Could you check a few things on this model? Use its own coordinates, in mm. A direction names the side the tool comes from. Coordinates: 2 decimals unless noted, no trailing zeros. Loops run counter-clockwise (first coordinate to the right, second up) from the corner with the lowest first, then second, coordinate; pieces in that order, holes last. Notation, with made-up numbers: M 29.5,31 L 34.5,31 A20 cw 34.5,62 Z; hole C -17,0 d10. An arc over 180 degrees is marked long. Return JSON: item names as keys, results as strings. Group by question number.
from build123d import *
from build123d.topology import SkipClean

# Parameters (mm, degrees)
BOSS_EXTRU_1_DEPTH           = 18
ENL_V_MAT_EXTRU_1_DEPTH      = 34.301651611
ENL_V_MAT_EXTRU_1_DEPTH_BACK = 34.301651611
ESQUISSE2_R                  = 2.85
ENL_V_MAT_EXTRU_2_DEPTH      = 34.301651611
ENL_V_MAT_EXTRU_2_DEPTH_BACK = 34.301651611
ESQUISSE3_R                  = 2.7
BOSS_EXTRU_2_DEPTH           = 3
BOSS_EXTRU_3_START           = -18
BOSS_EXTRU_3_DEPTH           = 3
CONG_1_R                     = 6
ESQUISSE6_R                  = 5
ESQUISSE6_R_2                = 3.1
BOSS_EXTRU_4_DEPTH           = 15
ESQUISSE7_R                  = 3.1
ESQUISSE7_R_2                = 2.7
BOSS_EXTRU_5_DEPTH           = 7


with BuildPart() as part:
    # Esquisse1 → Boss.-Extru.1 (new body)
    with BuildSketch(Plane.XY):
        Polygon((0, 0), (23, 0), (23, 16), (21.8, 16), (21.8, 3), (0, 3), align=None)
    extrude(amount=BOSS_EXTRU_1_DEPTH)

    # Esquisse2 → Enlèv. mat.-Extru.1 (cut, two sides: drawn at the far end of the back side and taken through both)
    with BuildSketch(Plane(origin=(23, 0, 0), x_dir=(0, 0, -1), z_dir=(1, 0, 0)).offset(-ENL_V_MAT_EXTRU_1_DEPTH_BACK)):
        with Locations((-9, 9)):
            Circle(ESQUISSE2_R)
    extrude(amount=ENL_V_MAT_EXTRU_1_DEPTH + ENL_V_MAT_EXTRU_1_DEPTH_BACK, mode=Mode.SUBTRACT)

    # Esquisse3 → Enlèv. mat.-Extru.2 (cut, two sides: drawn at the far end of the back side and taken through both)
    with BuildSketch(Plane.XZ.offset(-ENL_V_MAT_EXTRU_2_DEPTH_BACK)):
        with Locations((6, 9)):
            Circle(ESQUISSE3_R)
    extrude(amount=ENL_V_MAT_EXTRU_2_DEPTH + ENL_V_MAT_EXTRU_2_DEPTH_BACK, mode=Mode.SUBTRACT)

    # Esquisse4 → Boss.-Extru.2 (add)
    with BuildSketch(Plane.XY.offset(18)):
        Polygon((21.8, 3), (21.8, 16), (18.8, 3), align=None)
    extrude(amount=-BOSS_EXTRU_2_DEPTH)

    # Esquisse4<2> → Boss.-Extru.3 (add)
    with BuildSketch(Plane.XY.offset(18).offset(BOSS_EXTRU_3_START)):
        Polygon((21.8, 3), (21.8, 16), (18.8, 3), align=None)
    extrude(amount=BOSS_EXTRU_3_DEPTH)

    # Congé1
    cong_1_edges = [part.edges().sort_by_distance(p)[0] for p in [
        (0, 1.5, 18),
        (0, 1.5, 0),
    ]]
    fillet(cong_1_edges, radius=CONG_1_R)

    # Esquisse6 → Boss.-Extru.4 (add)
    with BuildSketch(Plane(origin=(0, 3, 0), x_dir=(1, 0, 0), z_dir=(0, 1, 0))):
        with Locations((6, -9)):
            Circle(ESQUISSE6_R)
        with Locations(Location((6, -9, 0), (0, 0, 180))):
            Circle(ESQUISSE6_R_2, mode=Mode.SUBTRACT)
    extrude(amount=BOSS_EXTRU_4_DEPTH)

    # Esquisse7 → Boss.-Extru.5 (add)
    with SkipClean():  # the faces are left unmerged after this step: merging them gives an invalid solid
        with BuildSketch(Plane(origin=(0, 3, 0), x_dir=(1, 0, 0), z_dir=(0, 1, 0))):
            with Locations(Location((6, -9, 0), (0, 0, 180))):
                Circle(ESQUISSE7_R)
            with Locations(Location((6, -9, 0), (0, 0, 180))):
                Circle(ESQUISSE7_R_2, mode=Mode.SUBTRACT)
        extrude(amount=BOSS_EXTRU_5_DEPTH)


solid = part.part
(1) If I drill on L1, parallel to X at y = 5.25, z = 9; L2, parallel to X at y = 2.05, z = 9; L3, parallel to Z at x = 21.75, y = 9.5, over which ranges is the centre line in solid material (lowest first)? Write a range as [from, to].
(2) Imagine slicing it at C-C, the plane x = 4.25. Write out the boundary of the cut face in (y, z), then the cut area to 3 significant figures.
(3) We'd pull the mould along Z, two halves only. Please class faces 1 (the face through (22.392, 10.926, 11.101)), 2 (the face through (0, 2, 9)), 3 (the face through (2, 10, 6)): +Z half, -Z half, draft (parallel to the pull), parting line (faces both ways), or undercut.
(4) Imagine slicing it at D-D, the plane y = 3.5. Write out the boundary of the cut face in (x, z), then the cut area to 3 significant figures.
(5) Will these pins go through, and if not, where does the flat tip stop? P1, Ø5, axis at x = 12, y = 8.5, coming from the +Z side; P2, Ø1.5, axis at x = 10, y = 16, coming from the -Z side; P3, Ø1, axis at x = 4, y = 6, coming from the -Z side.
(6) Imagine slicing it at B-B, the plane z = 9. Write out the boundary of the cut face in (x, y), then the cut area to 3 significant figures.
(7) For faces 4 (the face through (20.32, 9.59, 1.48)), 5 (the face through (21, 7, 15)), 6 (the face through (8.46, 13.944, 7.114)), 7 (the face through (22, 16, 9)), 8 (the face through (23, 6, 9)), which set-ups out of +Z, -Z, +X, -X, +Y, -Y let a thin tool reach every point of the face, with its end or its side?
(8) Imagine slicing it at A-A, the plane y = 12.75. Write out the boundary of the cut face in (x, z), then the cut area to 3 significant figures.
Checks:
{
 "1": {"L1": "[1, 3.3], [8.7, 11], [21.8, 23]", "L2": "[0, 3.3], [8.7, 23]", "L3": "[0, 3], [15, 18]"},
 "2": {"outline": "M 0,0.26 L 3,0.26 L 3,4.32 L 18,4.32 L 18,6.44 L 10,6.44 L 10,6.94 L 0,6.94 Z; M 0,11.06 L 10,11.06 L 10,11.56 L 18,11.56 L 18,13.68 L 3,13.68 L 3,17.74 L 0,17.74 Z", "area": "111 mm²"},
 "3": {"face 1": "undercut", "face 2": "draft", "face 3": "parting line"},
 "4": {"outline": "C 6,9 d10; M 18.92,0 L 23,0 L 23,18 L 18.92,18 L 18.92,15 L 21.8,15 L 21.8,3 L 18.92,3 Z; hole C 6,9 d5.4", "area": "94.5 mm²"},
 "5": {"P1": "z = 12.57", "P2": "z = 5.2", "P3": "z = 4.23"},
 "6": {"outline": "M 0,0 L 3.3,0 L 3.3,10 L 2.9,10 L 2.9,18 L 1,18 L 1,3 L 0,3 Z; M 8.7,0 L 23,0 L 23,6.15 L 21.8,6.15 L 21.8,3 L 11,3 L 11,18 L 9.1,18 L 9.1,10 L 8.7,10 Z; M 21.8,11.85 L 23,11.85 L 23,16 L 21.8,16 Z", "area": "124 mm²"},
 "7": {"face 4": "+Z, -Z, -X, +Y", "face 5": "-X, +Y", "face 6": "+Y", "face 7": "+Z, -Z, +X, +Y", "face 8": "+Z, -Z, +X, +Y, -Y"},
 "8": {"outline": "C 6,9 d10; M 21.05,0 L 23,0 L 23,18 L 21.05,18 L 21.05,15 L 21.8,15 L 21.8,3 L 21.05,3 Z; hole C 6,9 d6.2", "area": "74.4 mm²"}
}
